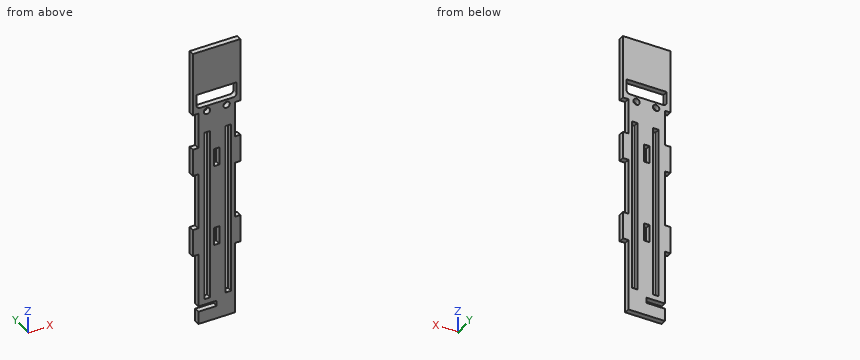
```python
from build123d import *

# Parameters (mm, degrees)
EXTRUDE_1_DEPTH     = 3
SKETCH_3_W          = 3
SKETCH_3_H          = 9.8
CUT_EXTRUDE_1_DEPTH = 10
SKETCH_4_W          = 26
SKETCH_4_H          = 35
EXTRUDE_2_DEPTH     = 3
SKETCH_5_W          = 22
SKETCH_5_H          = 8
CUT_EXTRUDE_2_DEPTH = 19
SKETCH_6_W          = 3
SKETCH_6_H          = 95
CUT_EXTRUDE_3_DEPTH = 25
FILLET_1_R          = 2
SKETCH_7_R          = 1.75
CUT_EXTRUDE_4_DEPTH = 10
SKETCH_8_R          = 1.75
SKETCH_8_W          = 3
SKETCH_8_H          = 95
CUT_EXTRUDE_5_DEPTH = 10


with BuildPart() as part:
    # Эскиз2 → Бобышка-Вытянуть1 (new body)
    with BuildSketch(Plane(origin=(0, 0, 0), x_dir=(1, 0, 0), z_dir=(0, 1, 0))):
        Polygon((-10, -60), (10, -60), (10, -40.4), (13, -40.4), (13, -25.4), (10, -25.4), (10, 5.4), (13, 5.4), (13, 20.4), (10, 20.4), (10, 60), (-10, 60), (-10, 53), (0, 53), (0, 50), (-10, 50), (-10, 20.4), (-13, 20.4), (-13, 5.4), (-10, 5.4), (-10, -25.4), (-13, -25.4), (-13, -40.4), (-10, -40.4), align=None)
    extrude(amount=EXTRUDE_1_DEPTH)

    # Эскиз3 → Вырез-Вытянуть1 (cut)
    with BuildSketch(Plane(origin=(0, 3, 0), x_dir=(1, 0, 0), z_dir=(0, 1, 0))):
        with Locations((0, 12.9)):
            Rectangle(SKETCH_3_W, SKETCH_3_H)
        with Locations((0, -32.1)):
            Rectangle(SKETCH_3_W, SKETCH_3_H)
    extrude(amount=-CUT_EXTRUDE_1_DEPTH, mode=Mode.SUBTRACT)

    # Эскиз4 → Бобышка-Вытянуть2 (add)
    with BuildSketch(Plane.XZ):
        with Locations((0, 77.5)):
            Rectangle(SKETCH_4_W, SKETCH_4_H)
    extrude(amount=-EXTRUDE_2_DEPTH)

    # Эскиз5 → Вырез-Вытянуть2 (cut)
    with BuildSketch(Plane(origin=(0, 0, 0), x_dir=(-1, 0, 0), z_dir=(0, -1, 0))):
        with Locations((0, -67)):
            Rectangle(SKETCH_5_W, SKETCH_5_H)
    extrude(amount=-CUT_EXTRUDE_2_DEPTH, mode=Mode.SUBTRACT)

    # Эскиз6 → Вырез-Вытянуть3 (cut)
    with BuildSketch(Plane.XZ):
        with Locations((6.5, 0.5)):
            Rectangle(SKETCH_6_W, SKETCH_6_H)
    extrude(amount=-CUT_EXTRUDE_3_DEPTH, mode=Mode.SUBTRACT)

    # Скругление1
    fillet_1_edges = [part.edges().sort_by_distance(p)[0] for p in [
        (-11, 1.5, 63),
        (11, 1.5, 63),
    ]]
    fillet(fillet_1_edges, radius=FILLET_1_R)

    # Эскиз7 → Вырез-Вытянуть4 (cut)
    with BuildSketch(Plane.XZ):
        with Locations(Location((5.5, 60, 0), (0, 0, 270))):
            Circle(SKETCH_7_R)
    extrude(amount=-CUT_EXTRUDE_4_DEPTH, mode=Mode.SUBTRACT)

    # Эскиз8 → Вырез-Вытянуть5 (cut)
    with BuildSketch(Plane.XZ):
        with Locations(Location((-5.229687219, 60, 0), (0, 0, 270))):
            Circle(SKETCH_8_R)
        with Locations((-5, 0.5)):
            Rectangle(SKETCH_8_W, SKETCH_8_H)
    extrude(amount=-CUT_EXTRUDE_5_DEPTH, mode=Mode.SUBTRACT)


solid = part.part
```
Could you check a few things on this model? Use its own coordinates, in mm. Give positions to 0.01 mm unless a question says otherwise; leave off trailing zeros. Order: outer loops, then holes, each group sorted by start corner. A loop starts at its lowest first (then second) coordinate and runs counter-clockwise, first axis right, second up.
Q1. I'm going to push flat-ended pins straight in: P1, Ø0.9, axis at y = 2, z = 19.5, coming from the +X side; P2, Ø1, axis at y = 0.5, z = 51, coming from the -X side; P3, Ø0.9, axis at x = -11, y = 1.5, coming from the -Z side. Where does each tip first touch, or does it pass through?
Q2. Suppose I cut it at B-B, the plane z = -14.5. Write out the boundary of the cut face in (x, y).
Q3. If I drill on line 1 along Z through (x, y) = (-8.5, 1.9); line 2 along Z through (x, y) = (-5, 1.45); line 3 along Z through (x, y) = (1, 2.85), over which ranges is the centre line in solid material (lowest first)?
Q4. Suppose I cut it at C-C, the plane y = 1.15. Count the separate pieces of the cut face and the enclosed holes in it, and give its area (3 significant figures).
Q5. Suppose I cut it at A-A, the plane z = 4. Write out the boundary of the cut face in (x, y), and give its area (3 significant figures).
Solution:
1. P1: stops at x = 10
1. P2: stops at x = -10
1. P3: stops at z = -20.4
2. outline: (-13, 0) - (-6.5, 0) - (-6.5, 3) - (-13, 3) - close; (-3.5, 0) - (-1.5, 0) - (-1.5, 3) - (-3.5, 3) - close; (1.5, 0) - (5, 0) - (5, 3) - (1.5, 3) - close; (8, 0) - (13, 0) - (13, 3) - (8, 3) - close
3. line 1: z = -60 to -53, -50 to 63, 71 to 95
3. line 2: z = -60 to -53, -50 to -47, 48 to 58.27, 61.73 to 63, 71 to 95
3. line 3: z = -60 to -17.8, -8 to 27.2, 37 to 63, 71 to 95
4. separate pieces: 1
4. enclosed holes: 7
4. area: 2,640 mm2
5. outline: (-10, 0) - (-6.5, 0) - (-6.5, 3) - (-10, 3) - close; (-3.5, 0) - (5, 0) - (5, 3) - (-3.5, 3) - close; (8, 0) - (10, 0) - (10, 3) - (8, 3) - close
5. area: 42.0 mm2
